from build123d import *

# Parameters (mm, degrees)
BASPROSKE_W             = 7.5
BASPROSKE_H             = 4.5
TOOTHCUT_DEPTH          = 10.836157786
TEETHCUTS_COUNT         = 16
TEETHCUTS_ANGLE         = 337.5
BORSKE_R                = 2.5
BORE_DEPTH              = 50.0000508
ESQUISSE4_R             = 6
BOSS_EXTRU_3_DEPTH      = 1
ESQUISSE5_R             = 6.027848577
ESQUISSE5_R_2           = 2.85
BOSS_EXTRU_4_DEPTH      = 1
ESQUISSE7_R             = 3.00711341
BOSS_EXTRU_6_DEPTH      = 8.5
ESQUISSE9_R             = 13.75
ESQUISSE9_R_2           = 5.5
BOSS_EXTRU_8_DEPTH      = 2
ESQUISSE10_R            = 1.5
ENL_V_MAT_EXTRU_3_DEPTH = 23.591480695
ESQUISSE11_R            = 3
ENL_V_MAT_EXTRU_4_DEPTH = 4
BOSS_EXTRU_9_START      = 4
ESQUISSE12_R            = 3
BOSS_EXTRU_9_DEPTH      = 4
ESQUISSE13_R            = 5.5
BOSS_EXTRU_10_DEPTH     = 2
ESQUISSE16_R            = 8
BOSS_EXTRU_11_DEPTH     = 1
ESQUISSE14_R            = 6
ENL_V_MAT_EXTRU_5_DEPTH = 1.5
ESQUISSE15_R            = 3.25
ENL_V_MAT_EXTRU_6_DEPTH = 4.5
ENL_V_START             = -4
ESQUISSE17_R            = 6.027848577
ENL_V_MAT_EXTRU_7_DEPTH = 4
ENL_V_MAT_EXTRU_8_DEPTH = 6


with BuildPart() as part:
    # BasProSke → Base-Revolve (revolve)
    with BuildSketch(Plane(origin=(0, 0, 0), x_dir=(1, 0, 0), z_dir=(0, 1, 0)), mode=Mode.PRIVATE) as base_revolve_sk:
        with Locations((3.75, 2.25)):
            Rectangle(BASPROSKE_W, BASPROSKE_H)
    revolve(base_revolve_sk.sketch.rotate(Axis((-10, 0, 0), (1, 0, 0)), 180), axis=Axis((-10, 0, 0), (1, 0, 0)))

    # TooCutSke → ToothCut (cut, through all)
    with BuildSketch(Plane(origin=(0, 0, 0), x_dir=(0, 0, -1), z_dir=(1, 0, 0))):
        with BuildLine():
            ThreePointArc((0.306025637, 3.360092902), (0, 3.374), (-0.306025637, 3.360092902))
            ThreePointArc((-0.306025637, 3.360092902), (-0.415941512, 3.953968919), (-0.738171669, 4.464789776))
            ThreePointArc((-0.738171669, 4.464789776), (0, 4.5254), (0.738171669, 4.464789776))
            ThreePointArc((0.738171669, 4.464789776), (0.415941512, 3.953968919), (0.306025637, 3.360092902))
        make_face()
    toothcut = extrude(amount=TOOTHCUT_DEPTH, mode=Mode.SUBTRACT)

    # TeethCuts: ToothCut ×16 about axis
    teethcuts_axis = Axis((-10, 0, 0), (1, 0, 0))
    for i in range(1, TEETHCUTS_COUNT):
        add(toothcut.rotate(teethcuts_axis, i * TEETHCUTS_ANGLE / (TEETHCUTS_COUNT - 1)), mode=Mode.SUBTRACT)

    # BorSke → Bore (cut, symmetric)
    with BuildSketch(Plane(origin=(0, 0, 0), x_dir=(0, 0, -1), z_dir=(1, 0, 0))):
        with Locations(Location((0, 0, 0), (0, 0, 180))):
            Circle(BORSKE_R)
    extrude(amount=BORE_DEPTH, both=True, mode=Mode.SUBTRACT)

    # Esquisse4 → Boss.-Extru.3 (add)
    with BuildSketch(Plane.ZY):
        Circle(ESQUISSE4_R)
    extrude(amount=BOSS_EXTRU_3_DEPTH)

    # Esquisse5 → Boss.-Extru.4 (add)
    with BuildSketch(Plane(origin=(7.5, 0, 0), x_dir=(0, 0, -1), z_dir=(1, 0, 0))):
        Circle(ESQUISSE5_R)
        Circle(ESQUISSE5_R_2, mode=Mode.SUBTRACT)
    extrude(amount=BOSS_EXTRU_4_DEPTH)

    # Esquisse7 → Boss.-Extru.6 (add)
    with BuildSketch(Plane(origin=(0, 0, 0), x_dir=(0, 0, -1), z_dir=(1, 0, 0))):
        Circle(ESQUISSE7_R)
    extrude(amount=BOSS_EXTRU_6_DEPTH)

    # Esquisse9 → Boss.-Extru.8 (add)
    with BuildSketch(Plane.ZY.offset(1)):
        Circle(ESQUISSE9_R)
        Circle(ESQUISSE9_R_2, mode=Mode.SUBTRACT)
    extrude(amount=BOSS_EXTRU_8_DEPTH)

    # Esquisse10 → Enlèv. mat.-Extru.3 (cut, through all)
    with BuildSketch(Plane.ZY.offset(3)):
        with Locations((0, 11.3)):
            Circle(ESQUISSE10_R)
        with Locations((0, -11.3)):
            Circle(ESQUISSE10_R)
    extrude(amount=-ENL_V_MAT_EXTRU_3_DEPTH, mode=Mode.SUBTRACT)

    # Esquisse11 → Enlèv. mat.-Extru.4 (cut)
    with BuildSketch(Plane.ZY.offset(1)):
        Circle(ESQUISSE11_R)
    extrude(amount=-ENL_V_MAT_EXTRU_4_DEPTH, mode=Mode.SUBTRACT)

    # Esquisse12 → Boss.-Extru.9 (add)
    with BuildSketch(Plane.ZY.offset(-3).offset(BOSS_EXTRU_9_START)):
        Circle(ESQUISSE12_R)
    extrude(amount=-BOSS_EXTRU_9_DEPTH)

    # Esquisse13 → Boss.-Extru.10 (add)
    with BuildSketch(Plane.ZY.offset(1)):
        Circle(ESQUISSE13_R)
    extrude(amount=BOSS_EXTRU_10_DEPTH)

    # Esquisse16 → Boss.-Extru.11 (add)
    with BuildSketch(Plane(origin=(-1, 0, 0), x_dir=(0, 0, -1), z_dir=(1, 0, 0))):
        with Locations(Location((0, 0, 0), (0, 0, 180))):
            Circle(ESQUISSE16_R)
    extrude(amount=BOSS_EXTRU_11_DEPTH)

    # Esquisse14 → Enlèv. mat.-Extru.5 (cut)
    with BuildSketch(Plane.ZY.offset(3)):
        Circle(ESQUISSE14_R)
    extrude(amount=-ENL_V_MAT_EXTRU_5_DEPTH, mode=Mode.SUBTRACT)

    # Esquisse15 → Enlèv. mat.-Extru.6 (cut)
    with BuildSketch(Plane.ZY.offset(1.5)):
        Circle(ESQUISSE15_R)
    extrude(amount=-ENL_V_MAT_EXTRU_6_DEPTH, mode=Mode.SUBTRACT)

    # Esquisse17 → Enlèv. mat.-Extru.7 (cut)
    with BuildSketch(Plane(origin=(8.5, 0, 0), x_dir=(0, 0, -1), z_dir=(1, 0, 0)).offset(ENL_V_START)):
        Circle(ESQUISSE17_R)
    extrude(amount=ENL_V_MAT_EXTRU_7_DEPTH, mode=Mode.SUBTRACT)

    # Esquisse18 → Enlèv. mat.-Extru.8 (cut)
    with BuildSketch(Plane(origin=(4.5, 0, 0), x_dir=(0, 0, -1), z_dir=(1, 0, 0))):
        with BuildLine():
            ThreePointArc((3.572076358, 0.117245432), (4.159283684, 0.287738258), (4.655535919, 0.644969227))
            ThreePointArc((4.655535919, 0.644969227), (4.609690818, 0.916924513), (4.547973386, 1.185722597))
            ThreePointArc((4.547973386, 1.185722597), (3.952789729, 1.325853469), (3.34503612, 1.258653786))
            ThreePointArc((3.34503612, 1.258653786), (3.301945449, 1.367710587), (3.255300351, 1.475295097))
            ThreePointArc((3.255300351, 1.475295097), (3.732564401, 1.857524443), (4.054335311, 2.377470333))
            ThreePointArc((4.054335311, 2.377470333), (3.907907178, 2.611180095), (3.748023133, 2.835898905))
            ThreePointArc((3.748023133, 2.835898905), (3.144519371, 2.737596024), (2.608744456, 2.442934375))
            ThreePointArc((2.608744456, 2.442934375), (2.527199636, 2.527199636), (2.442934375, 2.608744456))
            ThreePointArc((2.442934375, 2.608744456), (2.737596024, 3.144519371), (2.835898905, 3.748023133))
            ThreePointArc((2.835898905, 3.748023133), (2.611180095, 3.907907178), (2.377470333, 4.054335311))
            ThreePointArc((2.377470333, 4.054335311), (1.857524443, 3.732564401), (1.475295097, 3.255300351))
            ThreePointArc((1.475295097, 3.255300351), (1.367710587, 3.301945449), (1.258653786, 3.34503612))
            ThreePointArc((1.258653786, 3.34503612), (1.325853469, 3.952789729), (1.185722597, 4.547973386))
            ThreePointArc((1.185722597, 4.547973386), (0.916924513, 4.609690818), (0.644969227, 4.655535919))
            ThreePointArc((0.644969227, 4.655535919), (0.287738258, 4.159283684), (0.117245432, 3.572076358))
            ThreePointArc((0.117245432, 3.572076358), (0, 3.574), (-0.117245432, 3.572076358))
            ThreePointArc((-0.117245432, 3.572076358), (-0.287738258, 4.159283684), (-0.644969227, 4.655535919))
            ThreePointArc((-0.644969227, 4.655535919), (-0.916924513, 4.609690818), (-1.185722597, 4.547973386))
            ThreePointArc((-1.185722597, 4.547973386), (-1.325853469, 3.952789729), (-1.258653786, 3.34503612))
            ThreePointArc((-1.258653786, 3.34503612), (-1.367710587, 3.301945449), (-1.475295097, 3.255300351))
            ThreePointArc((-1.475295097, 3.255300351), (-1.857524443, 3.732564401), (-2.377470333, 4.054335311))
            ThreePointArc((-2.377470333, 4.054335311), (-2.611180095, 3.907907178), (-2.835898905, 3.748023133))
            ThreePointArc((-2.835898905, 3.748023133), (-2.737596024, 3.144519371), (-2.442934375, 2.608744456))
            ThreePointArc((-2.442934375, 2.608744456), (-2.527199636, 2.527199636), (-2.608744456, 2.442934375))
            ThreePointArc((-2.608744456, 2.442934375), (-3.144519371, 2.737596024), (-3.748023133, 2.835898905))
            ThreePointArc((-3.748023133, 2.835898905), (-3.907907178, 2.611180095), (-4.054335311, 2.377470333))
            ThreePointArc((-4.054335311, 2.377470333), (-3.732564401, 1.857524443), (-3.255300351, 1.475295097))
            ThreePointArc((-3.255300351, 1.475295097), (-3.301945449, 1.367710587), (-3.34503612, 1.258653786))
            ThreePointArc((-3.34503612, 1.258653786), (-3.952789729, 1.325853469), (-4.547973386, 1.185722597))
            ThreePointArc((-4.547973386, 1.185722597), (-4.609690818, 0.916924513), (-4.655535919, 0.644969227))
            ThreePointArc((-4.655535919, 0.644969227), (-4.159283684, 0.287738258), (-3.572076358, 0.117245432))
            ThreePointArc((-3.572076358, 0.117245432), (-3.574, 0), (-3.572076358, -0.117245432))
            ThreePointArc((-3.572076358, -0.117245432), (-4.159283684, -0.287738258), (-4.655535919, -0.644969227))
            ThreePointArc((-4.655535919, -0.644969227), (-4.609690818, -0.916924513), (-4.547973386, -1.185722597))
            ThreePointArc((-4.547973386, -1.185722597), (-3.952789729, -1.325853469), (-3.34503612, -1.258653786))
            ThreePointArc((-3.34503612, -1.258653786), (-3.301945449, -1.367710587), (-3.255300351, -1.475295097))
            ThreePointArc((-3.255300351, -1.475295097), (-3.732564401, -1.857524443), (-4.054335311, -2.377470333))
            ThreePointArc((-4.054335311, -2.377470333), (-3.907907178, -2.611180095), (-3.748023133, -2.835898905))
            ThreePointArc((-3.748023133, -2.835898905), (-3.144519371, -2.737596024), (-2.608744456, -2.442934375))
            ThreePointArc((-2.608744456, -2.442934375), (-2.527199636, -2.527199636), (-2.442934375, -2.608744456))
            ThreePointArc((-2.442934375, -2.608744456), (-2.737596024, -3.144519371), (-2.835898905, -3.748023133))
            ThreePointArc((-2.835898905, -3.748023133), (-2.611180095, -3.907907178), (-2.377470333, -4.054335311))
            ThreePointArc((-2.377470333, -4.054335311), (-1.857524443, -3.732564401), (-1.475295097, -3.255300351))
            ThreePointArc((-1.475295097, -3.255300351), (-1.367710587, -3.301945449), (-1.258653786, -3.34503612))
            ThreePointArc((-1.258653786, -3.34503612), (-1.325853469, -3.952789729), (-1.185722597, -4.547973386))
            ThreePointArc((-1.185722597, -4.547973386), (-0.916924513, -4.609690818), (-0.644969227, -4.655535919))
            ThreePointArc((-0.644969227, -4.655535919), (-0.287738258, -4.159283684), (-0.117245432, -3.572076358))
            ThreePointArc((-0.117245432, -3.572076358), (0, -3.574), (0.117245432, -3.572076358))
            ThreePointArc((0.117245432, -3.572076358), (0.287738258, -4.159283684), (0.644969227, -4.655535919))
            ThreePointArc((0.644969227, -4.655535919), (0.916924513, -4.609690818), (1.185722597, -4.547973386))
            ThreePointArc((1.185722597, -4.547973386), (1.325853469, -3.952789729), (1.258653786, -3.34503612))
            ThreePointArc((1.258653786, -3.34503612), (1.367710587, -3.301945449), (1.475295097, -3.255300351))
            ThreePointArc((1.475295097, -3.255300351), (1.857524443, -3.732564401), (2.377470333, -4.054335311))
            ThreePointArc((2.377470333, -4.054335311), (2.611180095, -3.907907178), (2.835898905, -3.748023133))
            ThreePointArc((2.835898905, -3.748023133), (2.737596024, -3.144519371), (2.442934375, -2.608744456))
            ThreePointArc((2.442934375, -2.608744456), (2.527199636, -2.527199636), (2.608744456, -2.442934375))
            ThreePointArc((2.608744456, -2.442934375), (3.144519371, -2.737596024), (3.748023133, -2.835898905))
            ThreePointArc((3.748023133, -2.835898905), (3.907907178, -2.611180095), (4.054335311, -2.377470333))
            ThreePointArc((4.054335311, -2.377470333), (3.732564401, -1.857524443), (3.255300351, -1.475295097))
            ThreePointArc((3.255300351, -1.475295097), (3.301945449, -1.367710587), (3.34503612, -1.258653786))
            ThreePointArc((3.34503612, -1.258653786), (3.952789729, -1.325853469), (4.547973386, -1.185722597))
            ThreePointArc((4.547973386, -1.185722597), (4.609690818, -0.916924513), (4.655535919, -0.644969227))
            ThreePointArc((4.655535919, -0.644969227), (4.159283684, -0.287738258), (3.572076358, -0.117245432))
            ThreePointArc((3.572076358, -0.117245432), (3.574, 0), (3.572076358, 0.117245432))
        make_face()
    extrude(amount=-ENL_V_MAT_EXTRU_8_DEPTH, mode=Mode.SUBTRACT)


solid = part.part
Source: CAD feature listing. Evaluate the final solid. Frame: model axes, mm. Coordinates: 2 decimals unless noted, no trailing zeros. Write each loop counter-clockwise with the first axis right and the second up, starting at its lowest first coordinate (ties: lowest second). Pieces come first, ordered by that corner, then holes. Notation, with made-up numbers: M 65,63 L 73,63 A20 ccw 73,96 Z; hole C 56,87.25 d5. An arc over 180 degrees is marked long. Use a Markdown table: item, result.
1) First-contact query: pin 1 Ø1 at (y, z) = (-3.5, 9) entering from +X; pin 2 Ø2 at (y, z) = (4, 2) entering from -X. Flat tips, straight axial feed; report the tip coordinate or a pass-through.
Conclusion:
| item | result |
|---|---|
| pin 1 | stops at x = -1 |
| pin 2 | stops at x = -1.5 |
2) Section B-B, the plane x = -2.55. Output: boundary loops of the cut face in (y, z).
Conclusion:
| item | result |
|---|---|
| outline | C 0,0 d27.5; hole C -11.3,0 d3; hole C 0,0 d12; hole C 11.3,0 d3 |
3) Section D-D, the plane y = -6.5. Output: boundary loops of the cut face in (x, z), then the cut area to 3 significant figures.
Conclusion:
| item | result |
|---|---|
| outline | M -3,-12.12 L -1,-12.12 L -1,-4.66 L 0,-4.66 L 0,4.66 L -1,4.66 L -1,12.12 L -3,12.12 Z |
| area | 57.8 mm^2 |
4) Mould query, pull axis Y, two halves, no side actions, for faces 1 (the cylindrical face through (-0.739, -3.738, 1.864)), 2 (the cylindrical face through (-1.986, -13.423, -2.981)), 3 (the cylindrical face through (-0.739, 1.326, 3.944)). Classes: pulls with the +Y half, pulls with the -Y half, needs draft (parallel to the pull), parting line crosses it, or undercut.
Conclusion:
| item | result |
|---|---|
| face 1 | undercut |
| face 2 | parting line crosses it |
| face 3 | undercut |
5) Ray query, L1, parallel to Y at x = -2.25, z = 0; L2, parallel to Y at x = -2.55, z = -0.5; L3, parallel to X at y = 10.25, z = 1.25. Return the intervals inside material, ascending.
Conclusion:
| item | result |
|---|---|
| L1 | y = -13.75 to -12.8, -9.8 to -6, 6 to 9.8, 12.8 to 13.75 |
| L2 | y = -13.74 to -12.71, -9.89 to -5.98, 5.98 to 9.89, 12.71 to 13.74 |
| L3 | x = -3 to -1 |
6) Section A-A, the plane y = -11.3. Output: boundary loops of the cut face in (x, z), then the cut area to 3 significant figures.
Conclusion:
| item | result |
|---|---|
| outline | M -3,-7.83 L -1,-7.83 L -1,-1.5 L -3,-1.5 Z; M -3,1.5 L -1,1.5 L -1,7.83 L -3,7.83 Z |
| area | 25.3 mm^2 |
7) Section C-C, the plane z = -5.25. Output: boundary loops of the cut face in (x, y), then the cut area to 3 significant figures.
Conclusion:
| item | result |
|---|---|
| outline | M -3,-12.71 L -1,-12.71 L -1,-6.04 L 0,-6.04 L 0,6.04 L -1,6.04 L -1,12.71 L -3,12.71 L -3,2.9 L -1.5,2.9 L -1.5,-2.9 L -3,-2.9 Z |
| area | 54.2 mm^2 |
